Autodesk Fusion 360 part; units mm, degrees
sketch "Sketch1" plane through (0, 0, 0) normal (0, 0, 1) x (1, 0, 0)
  circle A0 centre (0, 0) radius 12.5
  circle A1 centre (0, 0) radius 17.5
  line L0 (-9.525, 14.6807) -> (9.525, 14.6807)
  line L1 (-4.525, 11.6522) -> (-9.525, 11.6522)
  line L2 (-9.525, 11.6522) -> (-9.525, 24.6807)
  line L3 (-9.525, 24.6807) -> (-4.525, 24.6807)
  line L4 (-4.525, 24.6807) -> (-4.525, 11.6522)
  line L5 (4.525, 11.6522) -> (9.525, 11.6522)
  line L6 (9.525, 11.6522) -> (9.525, 24.6807)
  line L7 (9.525, 24.6807) -> (4.525, 24.6807)
  line L8 (4.525, 24.6807) -> (4.525, 11.6522)
  line L9 (0.0006, -27.5) -> (12.2475, -27.5)
  line L10 (12.2475, -27.5) -> (12.2475, -12.5)
  line L11 (12.2475, -12.5) -> (0.0006, -12.5)
  line L12 (0.0006, -12.5) -> (0.0006, -27.5)
  line L13 (-12.2462, -27.5) -> (-12.2462, -12.5)
  line L14 (0.0006, -27.5) -> (-12.2462, -27.5)
  line L15 (-12.2462, -12.5) -> (0.0006, -12.5)
  line L16 (12.2475, -27.5) -> (12.2475, -41)
  line L17 (12.2475, -41) -> (-12.2462, -27.5)
  dimension "d1" = 25
  dimension "d2" = 35
  dimension "d3" = 19.05
  dimension "d4" = 10
  dimension "d5" = 5
  dimension "d6" = 5
  dimension "d7" = 10
  dimension "d18" = 12.2468
  dimension "d19" = 15
  dimension "d27" = 13.5
extrude "Extrude1" add sketch "Sketch1" along normal blind 25 contours A0 A1 L5 L6 L11 | L0 L5 L6 L8 | A0 A1 L1 L2 L15 | A1 L11 L12 | A1 L12 L15 | L0 L1 L2 L4 | A1 L0 L8 | A1 L9 L10 L12 | A1 L12 L13 L14 | A1 L0 L4 | A1 L6 L7 L8 | L9 L14 L16 L17 | A1 L2 L3 L4
hole "Hole1" at (9.525, 19.6807, 19) direction (-1, 0, 0) diameter 5 depth 20 tip angle 180
hole "Hole2" at (-9.525, 19.6807, 6) direction (1, 0, 0) diameter 5 depth 20 tip angle 180
equation "d6 = d5"
equation "d7 = d4"
Build history of the part. All positions in model axes, mm. A direction names the side the tool comes from. Coordinates: 2 decimals unless noted, no trailing zeros. Order: outer loops, then holes, each group sorted by start corner. A loop starts at its lowest first (then second) coordinate and runs counter-clockwise, first axis right, second up. Notation, with made-up numbers: (-6.75, 75.5) - (41.25, 75.5) arc R18 ccw to (41.25, 84.5) - close; hole circle Ø3 at (11, 59). An arc over 180 degrees is marked (long way). Write item = value, one per line. Start each with the question number.
1) Saw through at C-C on z = 6. Write the cut outline in (x, y) (1 decimal).
2) Two-plate mould, pull along X, no slides. Class faces 1 (the face through (9.525, 20, 12)), 2 (the face through (-7.1, 19.6, 21.5)), 3 (the face through (0.48, -12.49, 12.32)), 4 (the face through (-17.433, 1.525, 12.325)): pulls with the +X half, pulls with the -X half, needs draft (parallel to the pull), parting line crosses it, or undercut.
3) Saw through at D-D on z = 10.25. Write the cut outline in (x, y) (1 decimal).
4) Flat gauge pins, fed straight in: pin 1 Ø4 at (y, z) = (-11.5, 10.5) entering from -X; pin 2 Ø6.5 at (y, z) = (19.68, 6) entering from -X (3 decimals); pin 3 Ø1 at (x, z) = (-1, 6.5) entering from -Y. Where does each tip first touch, or does it go through?
5) 3-axis set-ups, long thin cutter, end or side, ignore diameter. For faces 5 (the face through (12.248, -27, 12)), 6 (the face through (0, -15, 25)), 7 (the face through (-4.525, 18, 12)), 8 (the face through (-12.246, -20, 12)), 9 (the face through (-9.525, 20, 12)): which of +Z, -Z, +X, -X, +Y, -Y reach the whole face in a straight line?
6) Saw through at B-B on x = -6. Write the cut outline in (y, z), then the cut area to 3 significant figures.
7) Saw through at A-A on y = 0. Write the cut outline in (x, z).
8) Wall check: line 1 along Y through (x, z) = (-7.5, 19); line 2 along X through (y, z) = (12.5, 8.25) (3 decimals); line 3 along Y through (x, z) = (-6.5, 19). Give the ranges that are in metal, low to high. Write a range as from..to.
From the geometry:
q1.outline = (-12.2, -27.5) - (12.2, -41) - (12.2, -12.5) arc R17.5 ccw to (9.5, 14.7) - (9.5, 17.2) - (4.5, 17.2) - (4.5, 11.7) arc R12.5 cw (long way) to (-4.5, 11.7) - (-4.5, 17.2) - (-9.5, 17.2) - (-9.5, 14.7) arc R17.5 ccw to (-12.2, -12.5) - close; (-9.5, 22.2) - (-4.5, 22.2) - (-4.5, 24.7) - (-9.5, 24.7) - close; (4.5, 22.2) - (9.5, 22.2) - (9.5, 24.7) - (4.5, 24.7) - close
q2.face_1 = pulls with the +X half
q2.face_2 = needs draft
q2.face_3 = undercut
q2.face_4 = pulls with the -X half
q3.outline = (-12.2, -27.5) - (12.2, -41) - (12.2, -12.5) arc R17.5 ccw to (9.5, 14.7) - (9.5, 24.7) - (4.5, 24.7) - (4.5, 11.7) arc R12.5 cw (long way) to (-4.5, 11.7) - (-4.5, 24.7) - (-9.5, 24.7) - (-9.5, 14.7) arc R17.5 ccw to (-12.2, -12.5) - close
q4.pin_1 = -14.7
q4.pin_2 = -9.525
q4.pin_3 = -33.97
q5.face_5 = +Z, -Z, +X, -Y
q5.face_6 = +Z, +X, -X, +Y, -Y
q5.face_7 = +Z, -Z, +Y
q5.face_8 = +Z, -Z, -X, -Y
q5.face_9 = +Z, -Z, -X, +Y
q6.outline = (-30.94, 0) - (-10.97, 0) - (-10.97, 25) - (-30.94, 25) - close; (10.97, 0) - (24.68, 0) - (24.68, 25) - (10.97, 25) - close; hole circle Ø5 at (19.68, 6); hole circle Ø5 at (19.68, 19)
q6.area = 803 mm^2
q7.outline = (-17.5, 0) - (-12.5, 0) - (-12.5, 25) - (-17.5, 25) - close; (12.5, 0) - (17.5, 0) - (17.5, 25) - (12.5, 25) - close
q8.line_1 = -30.12..-10, 10..17.18, 22.18..24.68
q8.line_2 = -12.247..-4.525, 4.525..12.247
q8.line_3 = -30.67..-10.68, 10.68..17.18, 22.18..24.68
